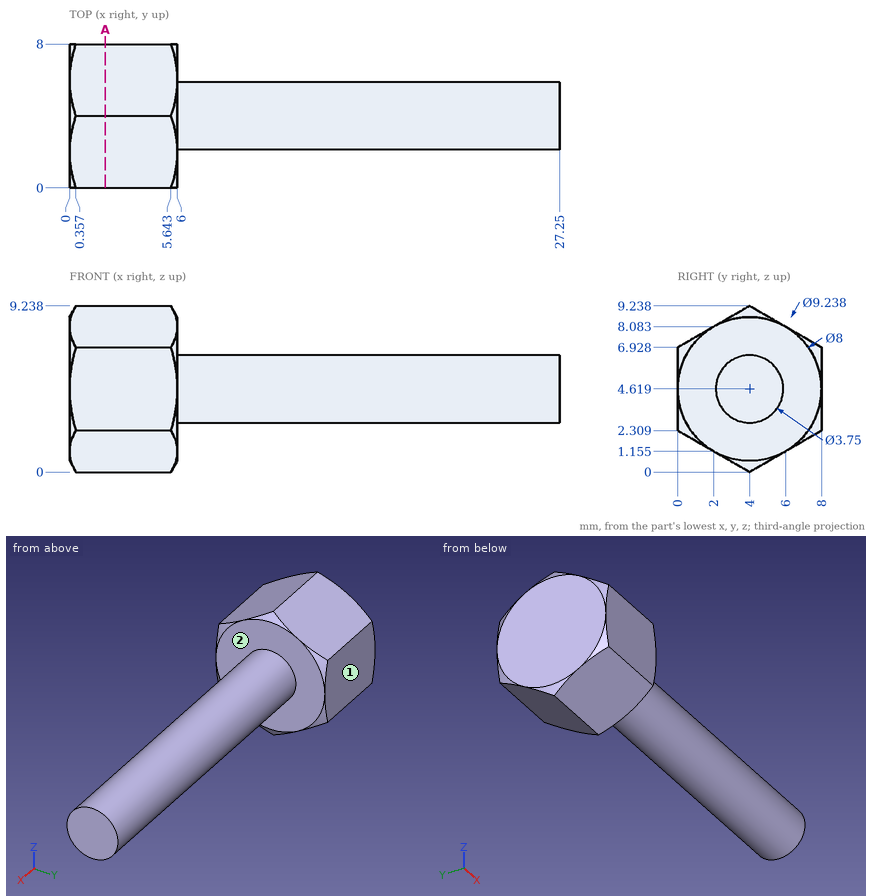
Check sheet for the drawn part. Datum: minimum x, y, z corner. Units: mm. A direction names the side the tool comes from. Coordinates: 2 decimals unless noted, no trailing zeros. Loops run counter-clockwise (first coordinate to the right, second up) from the corner with the lowest first, then second, coordinate; pieces in that order, holes last. Notation, with made-up numbers: (50, 25) -> (61, 25) arc R10 cw to (61, 35) -> close; hole circle Ø5 at (75.5, -21.5). An arc over 180 degrees is marked (long way). Answer in a Markdown table with one row per item.
1. Material ranges on line 1 along Y through (x, z) = (20.5, 4.5); line 2 along X through (y, z) = (4.25, 1.25); line 3 along Z through (x, y) = (25, 3.25), recorded low to high. Write a range as [from, to].
Check values:
| item | result |
|---|---|
| line 1 | y = [2.13, 5.87] |
| line 2 | x = [0, 6] |
| line 3 | z = [2.9, 6.34] |
2. Sectioned sample at A-A, the plane x = 2. Record the boundary of the cut face in (y, z).
Check values:
| item | result |
|---|---|
| outline | (0, 2.31) -> (4, 0) -> (8, 2.31) -> (8, 6.93) -> (4, 9.24) -> (0, 6.93) -> close |
3. Access from +Z, -Z, +X, -X, +Y, -Y to the whole of each face (thin tool, end or side, straight path). Record for the marked faces 1 and 2.
Check values:
| item | result |
|---|---|
| face 1 | +Z, -Z, +X, -X, +Y |
| face 2 | +X |
4. Go/stop test with flat-tipped pins: pin 1 (4 mm diameter, centred on x = 19, z = 3.5, fed in from -Y) (3 decimals); pin 2 (3 mm diameter, centred on x = 23.5, y = 4.5, fed in from +Z); pin 3 (2 mm diameter, centred on x = 16, z = 4, fed in from +Y) (3 decimals). Record where each tip stops, or that it passes through.
Check values:
| item | result |
|---|---|
| pin 1 | stops at y = 2.125 |
| pin 2 | stops at z = 6.49 |
| pin 3 | stops at y = 5.875 |
